from build123d import *

# Parameters (mm, degrees)
ESBO_O1_W                                    = 125
ESBO_O1_H                                    = 140
RESSALTO_EXTRUS_O1_DEPTH                     = 2.5
RESSALTO_EXTRUS_O2_DEPTH                     = 6
ESBO_O3_W                                    = 1.52
ESBO_O3_H                                    = 105
CORTE_EXTRUS_O1_DEPTH                        = 2
ESBO_O4_W                                    = 1.52
ESBO_O4_H                                    = 105
CORTE_EXTRUS_O2_DEPTH                        = 2
ESBO_O5_W                                    = 66
ESBO_O5_H                                    = 1.52
CORTE_EXTRUS_O3_DEPTH                        = 2
FILETE1_R                                    = 2
FILETE2_R                                    = 2
FILETE3_R                                    = 2
ESBO_O6_W                                    = 12
ESBO_O6_H                                    = 130
CORTE_EXTRUS_O4_DEPTH                        = 138.929522592
FILETE4_R                                    = 2
FILETE5_R                                    = 2
ESBO_O7_W                                    = 19.009766083
ESBO_O7_H                                    = 4
ESBO_O7_W_2                                  = 19
ESBO_O7_W_3                                  = 29.5
RESSALTO_EXTRUS_O3_DEPTH                     = 2
ESBO_O8_W                                    = 123
ESBO_O8_H                                    = 1.1
CORTE_EXTRUS_O5_DEPTH                        = 2
FILETE6_R                                    = 2
FUROS_GUIA_COM_3_0MM1_D                      = 3
FUROS_GUIA_COM_3_0MM1_CSINK_D                = 3.05
FUROS_GUIA_COM_3_0MM1_CSINK_ANGLE            = 90
REBAIXO_PARA_PARAFUSO_COM_CABE_A_PAN_2_COUNT = 2
REBAIXO_PARA_PARAFUSO_COM_CABE_A_PAN_2_PITCH = 101


with BuildPart() as part:
    # Esboço1 → Ressalto-extrusão1 (new body)
    with BuildSketch(Plane.XY):
        with Locations((10.140586838, -47.097815293)):
            Rectangle(ESBO_O1_W, ESBO_O1_H)
    extrude(amount=RESSALTO_EXTRUS_O1_DEPTH)

    # Esboço2 → Ressalto-extrusão2 (add)
    with BuildSketch(Plane.XY.offset(2.5)):
        Polygon((-24.859413162, -2.097815293), (-20.859413162, -2.097815293), (-20.859413162, -107.097815293), (41.140586838, -107.097815293), (41.140586838, -2.097815293), (45.140586838, -2.097815293), (45.140586838, -107.097815293), (45.140586838, -111.097815293), (-24.859413162, -111.097815293), (-24.859413162, -107.097815293), align=None)
    extrude(amount=RESSALTO_EXTRUS_O2_DEPTH)

    # Esboço3 → Corte-extrusão1 (cut)
    with BuildSketch(Plane.ZY.offset(-41.140586838)):
        with Locations((6.26, -54.597815293)):
            Rectangle(ESBO_O3_W, ESBO_O3_H)
    extrude(amount=-CORTE_EXTRUS_O1_DEPTH, mode=Mode.SUBTRACT)

    # Esboço4 → Corte-extrusão2 (cut)
    with BuildSketch(Plane(origin=(-20.859413162, 0, 0), x_dir=(0, 0, -1), z_dir=(1, 0, 0))):
        with Locations((-6.26, -54.597815293)):
            Rectangle(ESBO_O4_W, ESBO_O4_H)
    extrude(amount=-CORTE_EXTRUS_O2_DEPTH, mode=Mode.SUBTRACT)

    # Esboço5 → Corte-extrusão3 (cut)
    with BuildSketch(Plane(origin=(0, -107.097815293, 0), x_dir=(1, 0, 0), z_dir=(0, 1, 0))):
        with Locations((10.140586838, -6.26)):
            Rectangle(ESBO_O5_W, ESBO_O5_H)
    extrude(amount=-CORTE_EXTRUS_O3_DEPTH, mode=Mode.SUBTRACT)

    # Filete1
    filete1_edges = [part.edges().sort_by_distance(p)[0] for p in [
        (41.140586838, -107.097815293, 7.76),
        (-20.859413162, -107.097815293, 7.76),
        (41.140586838, -107.097815293, 4),
        (-20.859413162, -107.097815293, 4),
    ]]
    fillet(filete1_edges, radius=FILETE1_R)

    # Filete2
    filete2_edges = [part.edges().sort_by_distance(p)[0] for p in [
        (-24.859413162, -111.097815293, 5.5),
        (45.140586838, -111.097815293, 5.5),
    ]]
    fillet(filete2_edges, radius=FILETE2_R)

    # Filete3
    filete3_edges = [part.edges().sort_by_distance(p)[0] for p in [
        (10.140586838, -111.097815293, 2.5),
        (-24.273626724, -110.512028855, 2.5),
        (44.5548004, -110.512028855, 2.5),
        (-24.859413162, -55.597815293, 2.5),
        (45.140586838, -55.597815293, 2.5),
    ]]
    fillet(filete3_edges, radius=FILETE3_R)

    # Esboço6 → Corte-extrusão4 (cut, through all)
    with BuildSketch(Plane.XY.offset(2.5)):
        with Locations((-14.859413162, -42.097815293)):
            Rectangle(ESBO_O6_W, ESBO_O6_H)
        with Locations((35.140586838, -42.097815293)):
            Rectangle(ESBO_O6_W, ESBO_O6_H)
    extrude(amount=-CORTE_EXTRUS_O4_DEPTH, mode=Mode.SUBTRACT)

    # Filete4
    filete4_edges = [part.edges().sort_by_distance(p)[0] for p in [
        (-20.859413162, 22.902184707, 1.25),
        (-8.859413162, 22.902184707, 1.25),
        (41.140586838, 22.902184707, 1.25),
        (29.140586838, 22.902184707, 1.25),
    ]]
    fillet(filete4_edges, radius=FILETE4_R)

    # Filete5
    filete5_edges = [part.edges().sort_by_distance(p)[0] for p in [
        (-20.859413162, -107.097815293, 1.25),
        (-8.859413162, -107.097815293, 1.25),
        (41.140586838, -107.097815293, 1.25),
        (29.140586838, -107.097815293, 1.25),
    ]]
    fillet(filete5_edges, radius=FILETE5_R)

    # Esboço7 → Ressalto-extrusão3 (add)
    with BuildSketch(Plane.XY.offset(2.5)):
        with Locations((0.635703797, 20.902184707)):
            Rectangle(ESBO_O7_W, ESBO_O7_H)
        with Locations((19.640586838, 20.902184707)):
            Rectangle(ESBO_O7_W_2, ESBO_O7_H)
        with Locations((-37.609413162, 20.902184707)):
            Rectangle(ESBO_O7_W_3, ESBO_O7_H)
        with Locations((57.890586838, 20.902184707)):
            Rectangle(ESBO_O7_W_3, ESBO_O7_H)
    extrude(amount=RESSALTO_EXTRUS_O3_DEPTH)

    # Esboço8 → Corte-extrusão5 (cut)
    with BuildSketch(Plane.XY.offset(4.5)):
        with Locations((11.140586838, 20.902184707)):
            Rectangle(ESBO_O8_W, ESBO_O8_H)
    extrude(amount=-CORTE_EXTRUS_O5_DEPTH, mode=Mode.SUBTRACT)

    # Filete6
    # the kernel refuses this fillet: 2 mm, written as the material it adds along each edge
    with BuildSketch(Plane(origin=(43.140586838, 18.902184707, 2.5), x_dir=(0, 0, 1), z_dir=(1, 0, 0)), Plane(origin=(-52.359413162, 18.902184707, 2.5), x_dir=(0, 0, 1), z_dir=(1, 0, 0))) as filete6_piece_1:
        with BuildLine():
            CenterArc((FILETE6_R, FILETE6_R), FILETE6_R, 180, 90)
            Line((0, FILETE6_R), (0, 0))
            Line((0, 0), (FILETE6_R, 0))
        make_face()
    extrude(amount=29.5)
    with BuildSketch(Plane(origin=(29.140586838, 18.902184707, 2.5), x_dir=(0, 0, 1), z_dir=(-1, 0, 0))) as filete6_piece_2:
        with BuildLine():
            CenterArc((FILETE6_R, -FILETE6_R), FILETE6_R, 90, 90)
            Line((0, -FILETE6_R), (0, 0))
            Line((0, 0), (FILETE6_R, 0))
        make_face()
    extrude(amount=38)
    # the kernel refuses this fillet: 2 mm, written as the material it takes off along each edge
    with BuildSketch(Plane(origin=(29.140586838, 22.902184707, -2.307221131), x_dir=(-1, 0, 0), z_dir=(0, 0, 1))) as filete6_2_piece_1:
        with BuildLine():
            CenterArc((1.922888452, 2), FILETE6_R, 195.962014163, 74.037985837)
            Line((0, 1.45), (0, 0))
            Line((0, 0), (1.922888452, 0))
        make_face()
    extrude(amount=11.614442262, mode=Mode.SUBTRACT)
    with BuildSketch(Plane(origin=(-8.869179245, 22.902184707, -2.307221131), x_dir=(1, 0, 0), z_dir=(0, 0, 1))) as filete6_2_piece_2:
        with BuildLine():
            CenterArc((1.922888452, -2), FILETE6_R, 90, 74.037985837)
            Line((0, -1.45), (0, 0))
            Line((0, 0), (1.922888452, 0))
        make_face()
    extrude(amount=11.614442262, mode=Mode.SUBTRACT)

    # Furos-guia com Ø3.0mm1 (through all)
    with Locations(Plane.XY.offset(2.5)):
        with Locations((-44.109413162, -27.097815293), (-44.109413162, -67.097815293), (64.390586838, -27.094030717), (64.390586838, -67.094030814)):
            CounterSinkHole(FUROS_GUIA_COM_3_0MM1_D / 2, FUROS_GUIA_COM_3_0MM1_CSINK_D / 2, counter_sink_angle=FUROS_GUIA_COM_3_0MM1_CSINK_ANGLE)

    # Esboço14 → Rebaixo para parafuso com cabeça panela de M31 (revolve, cut)
    with BuildSketch(Plane(origin=(-40.359413162, -108.297815293, 0), x_dir=(0, 1, 0), z_dir=(1, 0, 0))):
        Polygon((0, 0), (0, 8.5), (1.7, 8.5), (1.7, 1.5), (3.5, 1.5), (3.5, 0.025), (3.525, 0), align=None)
    rebaixo_para_parafuso_com_cabe_a_panela = revolve(axis=Axis((-40.359413162, -108.297815293, -6.35), (0, 0, 1)), mode=Mode.SUBTRACT)

    # Rebaixo para parafuso com cabe_a pan 2: Rebaixo para parafuso com cabeça panela de M31 ×2
    with Locations(*[(i * REBAIXO_PARA_PARAFUSO_COM_CABE_A_PAN_2_PITCH, 0, 0) for i in range(1, REBAIXO_PARA_PARAFUSO_COM_CABE_A_PAN_2_COUNT)]):
        add(rebaixo_para_parafuso_com_cabe_a_panela, mode=Mode.SUBTRACT)


solid = part.part
Design review of the part built by this model. Coordinates are the model's own, in mm. A direction names the side the tool comes from. Coordinates: 2 decimals unless noted, no trailing zeros. Order: outer loops, then holes, each group sorted by start corner. A loop starts at its lowest first (then second) coordinate and runs counter-clockwise, first axis right, second up.
Item 1: The part is to be moulded in two halves that separate along X. For faces 4 (the flat face through (-39, -107, 1.5)), 5 (the flat face through (45.141, -56, 6)), 6 (the flat face through (-38, 22, 4.5)), say which applies: pulls with the +X half, pulls with the -X half, needs draft (parallel to the pull), parting line crosses it, or undercut.
Item 2: For faces 1 (the flat face through (29.141, -41, 1)), 2 (the cylindrical face through (-39.019, -105.065, 0.752)), 3 (the flat face through (11, -111.098, 6)), list the 3-axis set-ups (+Z, -Z, +X, -X, +Y, -Y) from which the entire face can be reached by the end or side of a thin tool; tool diameter is ignored.
Item 3: Take a section at C-C, the plane y = 1.5. Write out the cut boundary in (x, z), then the cut area to 4 significant figures.
Item 4: For line 1 (X direction, y = -101, z = 1.5); line 2 (Y direction, x = 22.5, z = 5.75); line 3 (Z direction, x = 12, y = 15.5), list the stretches that pass through material, from the lowest coordinate up.
Item 5: Take a section at B-B, the plane x = 20. Write out the cut boundary in (y, z).
Item 6: Take a section at D-D, the plane x = -28.5. Write out the cut boundary in (y, z), then the cut area to 3 significant figures.
Item 7: Take a section at A-A, the plane y = -39.5. Write out the cut boundary in (x, z).
Item 8: For pin 1 Ø1.6 at (y, z) = (-60.5, 7.5) entering from -X; pin 2 Ø0.6 at (x, z) = (15, 4) entering from -Y; pin 3 Ø0.5 at (y, z) = (-43.5, 6.5) entering from +X, all flat-tipped, find the tip position at first contact; note any pin that passes through.
The answers:
1. face 4: undercut
1. face 5: pulls with the +X half
1. face 6: needs draft
2. face 1: +Z, -Z, +Y
2. face 2: -Z
2. face 3: +Z, +X, -X, -Y
3. outline: (-52.36, 0) - (-20.86, 0) - (-20.86, 2.5) - (-52.36, 2.5) - close; (-8.86, 0) - (29.14, 0) - (29.14, 2.5) - (-8.86, 2.5) - close; (41.14, 0) - (72.64, 0) - (72.64, 2.5) - (41.14, 2.5) - close
3. area: 252.5 mm2
4. line 1: x = -52.36 to -20.86, -8.86 to 29.14, 41.14 to 72.64
4. line 2: y = -111.1 to -109.1
4. line 3: z = 0 to 2.5
5. outline: (-117.1, 0) - (22.9, 0) - (22.9, 4.5) - (21.45, 4.5) - (21.45, 2.5) - (20.35, 2.5) - (20.35, 4.5) - (18.9, 4.5) arc R2 cw to (16.9, 2.5) - (-107.1, 2.5) - (-107.1, 5.5) - (-109.1, 5.5) - (-109.1, 7.02) - (-107.1, 7.02) - (-107.1, 8.5) - (-111.1, 8.5) - (-111.1, 4.5) arc R2 cw to (-113.1, 2.5) - (-117.1, 2.5) - close
6. outline: (-117.1, 0) - (22.9, 0) - (22.9, 4.5) - (21.45, 4.5) - (21.45, 2.5) - (20.35, 2.5) - (20.35, 4.5) - (18.9, 4.5) arc R2 cw to (16.9, 2.5) - (-117.1, 2.5) - close
6. area: 357 mm2
7. outline: (-52.36, 0) - (-20.86, 0) - (-20.86, 5.5) - (-22.86, 5.5) - (-22.86, 7.02) - (-20.86, 7.02) - (-20.86, 8.5) - (-24.86, 8.5) - (-24.86, 4.5) arc R2 cw to (-26.86, 2.5) - (-52.36, 2.5) - close; (-8.86, 0) - (29.14, 0) - (29.14, 2.5) - (-8.86, 2.5) - close; (41.14, 0) - (72.64, 0) - (72.64, 2.5) - (47.14, 2.5) arc R2 cw to (45.14, 4.5) - (45.14, 8.5) - (41.14, 8.5) - (41.14, 7.02) - (43.14, 7.02) - (43.14, 5.5) - (41.14, 5.5) - close
8. pin 1: stops at x = -24.86
8. pin 2: stops at y = -111.26
8. pin 3: stops at x = 45.14
